The model under review builds one solid part; all positions refer to its coordinate system, in mm. A direction names the side the tool comes from. Give positions to 0.01 mm unless a question says otherwise; leave off trailing zeros. Loops run counter-clockwise (first coordinate to the right, second up) from the corner with the lowest first, then second, coordinate; pieces in that order, holes last. Notation, with made-up numbers: M -8,23 L 17,23 A21 ccw 17,40 Z; hole C -21.75,87 d11. An arc over 180 degrees is marked long. Return JSON: item names as keys, results as strings.
Autodesk Inventor part; units mm, degrees
ref_plane "slider_ip1_XY" through (0, 0, 0) normal (1, 0, 0) x (0, 0, -1)
ref_plane "slider_ip1_YZ" through (0, 0, 0) normal (0, 0, -1) x (0, 1, 0)
ref_plane "slider_ip1_ZX" through (0, 0, 0) normal (0, 1, 0) x (1, 0, 0)
sketch "Sketch_1" plane through (0, 0, 12) normal (0, 0, 1) x (1, 0, 0)
  arc A0 (0, -19) -> (2, -21) centre (2, -19) ccw
  line L0 (2, -21) -> (64, -21)
  arc A1 (64, -21) -> (66, -19) centre (64, -19) ccw
  line L1 (66, -19) -> (66, 19)
  arc A2 (66, 19) -> (64, 21) centre (64, 19) ccw
  line L2 (64, 21) -> (2, 21)
  arc A3 (2, 21) -> (0, 19) centre (2, 19) ccw
  line L3 (0, 19) -> (0, -19)
extrude "Extrusion1" add sketch "Sketch_1" against normal blind 2.3
sketch "Sketch_6" plane through (0, 0, 9.7) normal (0, 0, 1) x (1, 0, 0)
  line L0 (3, 10.9) -> (3, -10.9)
  line L1 (3, -10.9) -> (63, -10.9)
  line L2 (63, -10.9) -> (63, 10.9)
  line L3 (63, 10.9) -> (3, 10.9)
extrude "Extrusion2" add sketch "Sketch_6" against normal blind 5
sketch "Sketch_2_ALT_Drilling_1" plane through (13, 0, 0) normal (1, 0, 0) x (0, 0, -1)
  line L0 (-12, 17) -> (-9.7, 17)
  line L1 (-9.7, 17) -> (-9.7, 15)
  line L2 (-9.7, 15) -> (-10.079, 15.379)
  line L3 (-10.079, 15.379) -> (-11.621, 15.379)
  line L4 (-11.621, 15.379) -> (-12, 15)
  line L5 (-12, 15) -> (-12, 17)
  line L6 (-12, 17) -> (-9.7, 17)
revolve "Revolution1" cut sketch "Sketch_2_ALT_Drilling_1" angle 360 about axis through (13, 17, 12) along (0, 0, 1)
thread "Thread1"
sketch "Sketch_3_ALT_Drilling_2" plane through (13, 0, 0) normal (1, 0, 0) x (0, 0, -1)
  line L0 (-12, -17) -> (-9.7, -17)
  line L1 (-9.7, -17) -> (-9.7, -19)
  line L2 (-9.7, -19) -> (-10.079, -18.621)
  line L3 (-10.079, -18.621) -> (-11.621, -18.621)
  line L4 (-11.621, -18.621) -> (-12, -19)
  line L5 (-12, -19) -> (-12, -17)
  line L6 (-12, -17) -> (-9.7, -17)
revolve "Revolution2" cut sketch "Sketch_3_ALT_Drilling_2" angle 360 about axis through (13, -17, 12) along (0, 0, 1)
thread "Thread2"
sketch "Sketch_4_ALT_Drilling_3" plane through (53, 0, 0) normal (1, 0, 0) x (0, 0, -1)
  line L0 (-12, 17) -> (-9.7, 17)
  line L1 (-9.7, 17) -> (-9.7, 15)
  line L2 (-9.7, 15) -> (-10.079, 15.379)
  line L3 (-10.079, 15.379) -> (-11.621, 15.379)
  line L4 (-11.621, 15.379) -> (-12, 15)
  line L5 (-12, 15) -> (-12, 17)
  line L6 (-12, 17) -> (-9.7, 17)
revolve "Revolution3" cut sketch "Sketch_4_ALT_Drilling_3" angle 360 about axis through (53, 17, 12) along (0, 0, 1)
thread "Thread3"
sketch "Sketch_5_ALT_Drilling_4" plane through (53, 0, 0) normal (1, 0, 0) x (0, 0, -1)
  line L0 (-12, -17) -> (-9.7, -17)
  line L1 (-9.7, -17) -> (-9.7, -19)
  line L2 (-9.7, -19) -> (-10.079, -18.621)
  line L3 (-10.079, -18.621) -> (-11.621, -18.621)
  line L4 (-11.621, -18.621) -> (-12, -19)
  line L5 (-12, -19) -> (-12, -17)
  line L6 (-12, -17) -> (-9.7, -17)
revolve "Revolution4" cut sketch "Sketch_5_ALT_Drilling_4" angle 360 about axis through (53, -17, 12) along (0, 0, 1)
thread "Thread4"
sketch "Sketch_8_ALT_Drilling_5" plane through (7, 0, 0) normal (1, 0, 0) x (0, 0, -1)
  line L0 (-10.85, 6) -> (-12, 6)
  line L1 (-12, 6) -> (-12, 8.75)
  line L2 (-12, 8.75) -> (-10.85, 8.75)
  line L3 (-10.85, 8.75) -> (-10.85, 6)
  line L4 (-10.85, 6) -> (-12, 6)
revolve "Revolution5" cut sketch "Sketch_8_ALT_Drilling_5" angle 360 about axis through (7, 6, 10.85) along (0, 0, -1)
sketch "Sketch_9_ALT_Drilling_6" plane through (7, 0, 0) normal (1, 0, 0) x (0, 0, -1)
  line L0 (-10.85, -6) -> (-12, -6)
  line L1 (-12, -6) -> (-12, -3.25)
  line L2 (-12, -3.25) -> (-10.85, -3.25)
  line L3 (-10.85, -3.25) -> (-10.85, -6)
  line L4 (-10.85, -6) -> (-12, -6)
revolve "Revolution6" cut sketch "Sketch_9_ALT_Drilling_6" angle 360 about axis through (7, -6, 10.85) along (0, 0, -1)
sketch "Sketch_10_ALT_Drilling_7" plane through (59, 0, 0) normal (1, 0, 0) x (0, 0, -1)
  line L0 (-10.85, 6) -> (-12, 6)
  line L1 (-12, 6) -> (-12, 8.75)
  line L2 (-12, 8.75) -> (-10.85, 8.75)
  line L3 (-10.85, 8.75) -> (-10.85, 6)
  line L4 (-10.85, 6) -> (-12, 6)
revolve "Revolution7" cut sketch "Sketch_10_ALT_Drilling_7" angle 360 about axis through (59, 6, 10.85) along (0, 0, -1)
sketch "Sketch_11_ALT_Drilling_8" plane through (59, 0, 0) normal (1, 0, 0) x (0, 0, -1)
  line L0 (-10.85, -6) -> (-12, -6)
  line L1 (-12, -6) -> (-12, -3.25)
  line L2 (-12, -3.25) -> (-10.85, -3.25)
  line L3 (-10.85, -3.25) -> (-10.85, -6)
  line L4 (-10.85, -6) -> (-12, -6)
revolve "Revolution8" cut sketch "Sketch_11_ALT_Drilling_8" angle 360 about axis through (59, -6, 10.85) along (0, 0, -1)
ref_plane "slider_ip1_XY" through (0, 0, 0) normal (1, 0, 0) x (0, 0, -1)
ref_plane "slider_ip1_YZ" through (0, 0, 0) normal (0, 0, -1) x (0, 1, 0)
ref_plane "slider_ip1_ZX" through (0, 0, 0) normal (0, 1, 0) x (1, 0, 0)
properties part number "FBW2560R+640 L Slider"
1) Consider section A-A on y = -10. Write out the cut boundary in (x, z), then the cut area to 3 significant figures.
From the geometry:
{"outline": "M 0,9.7 L 3,9.7 L 3,4.7 L 63,4.7 L 63,9.7 L 66,9.7 L 66,12 L 0,12 Z", "area": "452 mm²"}
2) Consider section C-C on y = -17. Write out the cut boundary in (x, z).
From the geometry:
{"outline": "M 0,9.7 L 11,9.7 L 11.38,10.08 L 11.38,11.62 L 11,12 L 0,12 Z; M 14.62,10.08 L 15,9.7 L 51,9.7 L 51.38,10.08 L 51.38,11.62 L 51,12 L 15,12 L 14.62,11.62 Z; M 54.62,10.08 L 55,9.7 L 66,9.7 L 66,12 L 55,12 L 54.62,11.62 Z"}
3) Consider section D-D on z = 8. Write out the cut boundary in (x, y), then the cut area to 3 significant figures.
From the geometry:
{"outline": "M 3,-10.9 L 63,-10.9 L 63,10.9 L 3,10.9 Z", "area": "1,310 mm²"}
4) Wall thickness on L1, parallel to X at y = 17, z = 10.9; L2, parallel to X at y = -6, z = 11.4; L3, parallel to Y at x = 43, z = 9: over which ranges is each line inside the solid? List them lowest first. Write a range as from..to.
From the geometry:
{"L1": "0..11.38, 14.62..51.38, 54.62..66", "L2": "0..4.25, 9.75..56.25, 61.75..66", "L3": "-10.9..10.9"}
5) Tool access review of faces 5 (the face through (33, 0, 12)), 6 (the face through (63, 0, 7)), 7 (the face through (59, -6, 10.85)): name each direction out of +Z, -Z, +X, -X, +Y, -Y from which nothing blocks a thin tool from reaching the whole face with its end or side.
From the geometry:
{"face 5": "+Z, +X, -X, +Y, -Y", "face 6": "-Z, +X, +Y, -Y", "face 7": "+Z"}
6) Consider section B-B on x = 29. Write out the cut boundary in (y, z).
From the geometry:
{"outline": "M -21,9.7 L -10.9,9.7 L -10.9,4.7 L 10.9,4.7 L 10.9,9.7 L 21,9.7 L 21,12 L -21,12 Z"}
7) The part is to be moulded in two halves that separate along X. For faces 1 (the face through (66, 0, 11)), 2 (the face through (13.487, 15.454, 10.861)), 3 (the face through (0.6, 20.43, 10.87)), 4 (the face through (33, 21, 11)), say which applies: released by +X, released by -X, zero draft, split by the parting line, or undercut.
From the geometry:
{"face 1": "released by +X", "face 2": "undercut", "face 3": "released by -X", "face 4": "zero draft"}
8) Insertion check: pin 1 (1.5 mm diameter, centred on x = 29, z = 7, fed in from -Y); pin 2 (2.5 mm diameter, centred on y = 2.5, z = 6.5, fed in from +X); pin 3 (3 mm diameter, centred on x = 59, y = -6.5, fed in from +Z). Each pin has a flat end and moves straight along its axis. Give the tip position at first contact, or say it passes through.
From the geometry:
{"pin 1": "y = -10.9", "pin 2": "x = 63", "pin 3": "z = 10.85"}
